Build history of the part. All positions in model axes, mm. Face numbers are marked on the shaded views. Coordinates: 2 decimals unless noted, no trailing zeros. Write each loop counter-clockwise with the first axis right and the second up, starting at its lowest first coordinate (ties: lowest second). Pieces come first, ordered by that corner, then holes.
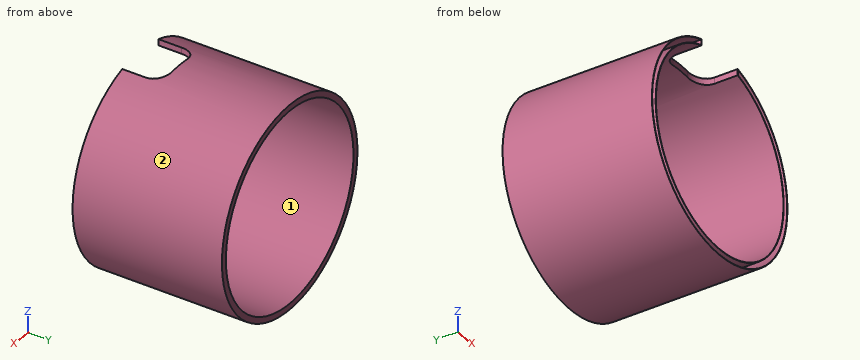
from build123d import *

# Parameters (mm, degrees)
SKETCH1_R           = 855
SKETCH1_R_2         = 805
BOSS_EXTRUDE1_DEPTH = 1300
CUT_EXTRUDE1_DEPTH  = 2646
CUT_EXTRUDE2_START  = -50
SKETCH3_R           = 855
CUT_EXTRUDE2_DEPTH  = 50
SHELL1_T            = -3


with BuildPart() as part:
    # Sketch1 → Boss-Extrude1 (new body)
    with BuildSketch(Plane(origin=(0, 0, 0), x_dir=(1, 0, 0), z_dir=(0, 1, 0))):
        with Locations(Location((0, 0, 0), (0, 0, 270))):
            Circle(SKETCH1_R)
        with Locations(Location((0, 0, 0), (0, 0, 270))):
            Circle(SKETCH1_R_2, mode=Mode.SUBTRACT)
    extrude(amount=BOSS_EXTRUDE1_DEPTH)

    # Sketch2 → Cut-Extrude1 (cut)
    with BuildSketch(Plane.XY):
        with BuildLine():
            Line((92.561405604, 330), (-92.561405604, 330))
            ThreePointArc((-92.561405604, 330), (-188.020821064, 290.45941546), (-227.561405604, 195))
            Line((-227.561405604, 195), (-227.561405604, -45))
            ThreePointArc((-227.561405604, -45), (-188.020821064, -140.45941546), (-92.561405604, -180))
            Line((-92.561405604, -180), (92.561405604, -180))
            ThreePointArc((92.561405604, -180), (188.020821064, -140.45941546), (227.561405604, -45))
            Line((227.561405604, -45), (227.561405604, 195))
            ThreePointArc((227.561405604, 195), (188.020821064, 290.45941546), (92.561405604, 330))
        make_face()
    extrude(amount=CUT_EXTRUDE1_DEPTH, mode=Mode.SUBTRACT)

    # Sketch3 → Cut-Extrude2 (cut)
    with BuildSketch(Plane(origin=(0, 1300, 0), x_dir=(1, 0, 0), z_dir=(0, 1, 0)).offset(CUT_EXTRUDE2_START)):
        with Locations(Location((0, 0, 0), (0, 0, 254.56448344))):
            Circle(SKETCH3_R)
    extrude(amount=CUT_EXTRUDE2_DEPTH, mode=Mode.SUBTRACT)

    # Shell1
    shell1_openings = [part.faces().sort_by_distance(p)[0] for p in [
        (251.527382632, 0, 798.163487829),
    ]]
    offset(amount=SHELL1_T, openings=shell1_openings)


solid = part.part
(1) Slice it at C-C, the plane y = 142.5. List the corners of the cut face in (x, z), and give its area (3 significant figures).
(2) Slice it at B-B, the plane z = 0. List the corners of the cut face in (x, y), and give its area (3 significant figures).
(3) Slice it at A-A, the plane x = 0. List the corners of the cut face in (y, z).
(4) Flat gauge pins, fed straight in: P1, Ø8, axis at y = 658.5, z = 371.5, coming from the -X side; P2, Ø8, axis at y = 802, z = 365, coming from the -X side; P3, Ø5, axis at y = 362, z = -252.5, coming from the +X side. Where does each tip first touch, or does it go through?
(5) Two-plate mould, pull along X, no slides. Class the marked faces 1 and 2: pulls with the +X half, pulls with the -X half, needs draft (parallel to the pull), parting line crosses it, or undercut.
(6) Slice it at D-D, the plane x = 491.5. List the corners of the cut face in (y, z).
(7) Probe L1, parallel to Z at x = 0, y = 934. List the from-to ranges inside material, lowest first.
Results:
1. outline: (-227.56, 772.17) - (-227.56, 824.16) arc R855 ccw (long way) to (227.56, 824.16) - (227.56, 772.17) arc R805 cw (long way) to start; hole (-230.56, 774.41) - (-230.56, 820.21) arc R852 ccw (long way) to (230.56, 820.21) - (230.56, 774.41) arc R808 cw (long way) to start
1. area: 28,800 mm2
2. outline: (-855, 0) - (-852, 0) - (-852, 1247) - (-808, 1247) - (-808, 0) - (-805, 0) - (-805, 1250) - (-855, 1250) - close; (805, 0) - (808, 0) - (808, 1247) - (852, 1247) - (852, 0) - (855, 0) - (855, 1250) - (805, 1250) - close
2. area: 15,300 mm2
3. outline: (0, -855) - (1250, -855) - (1250, -805) - (0, -805) - (0, -808) - (1247, -808) - (1247, -852) - (0, -852) - close; (330, 805) - (1250, 805) - (1250, 855) - (330, 855) - close; hole (333, 808) - (1247, 808) - (1247, 852) - (333, 852) - close
4. P1: stops at x = -771.99
4. P2: stops at x = -775.05
4. P3: stops at x = 817.63
5. face 1: undercut
5. face 2: parting line crosses it
6. outline: (0, -699.61) - (1250, -699.61) - (1250, -637.54) - (0, -637.54) - (0, -641.32) - (1247, -641.32) - (1247, -695.94) - (0, -695.94) - close; (0, 637.54) - (1250, 637.54) - (1250, 699.61) - (0, 699.61) - (0, 695.94) - (1247, 695.94) - (1247, 641.32) - (0, 641.32) - close
7. L1: z = -855 to -852, -808 to -805, 805 to 808, 852 to 855
